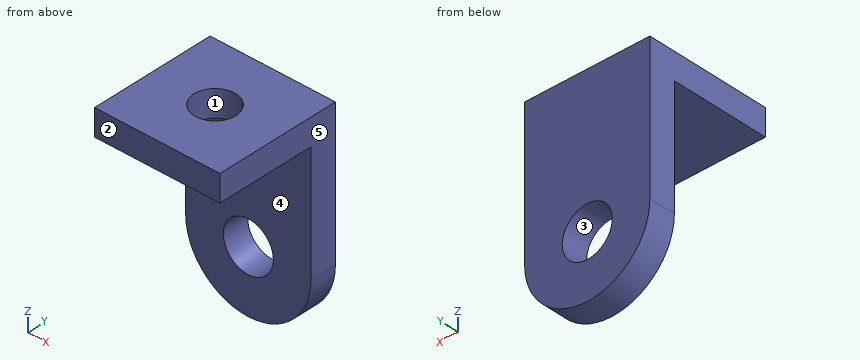
```python
from build123d import *

# Parameters (mm, degrees)
SKETCH1_W           = 15
SKETCH1_H           = 15
SKETCH1_R           = 2.5
BOSS_EXTRUDE1_DEPTH = 3.175
SKETCH2_R           = 3
BOSS_EXTRUDE2_DEPTH = 3.175


with BuildPart() as part:
    # Sketch1 → Boss-Extrude1 (new body)
    with BuildSketch(Plane.XY):
        with Locations((0, -7.5)):
            Rectangle(SKETCH1_W, SKETCH1_H)
        with Locations((0, -7.5)):
            Circle(SKETCH1_R, mode=Mode.SUBTRACT)
    extrude(amount=BOSS_EXTRUDE1_DEPTH)

    # Sketch2 → Boss-Extrude2 (add)
    with BuildSketch(Plane(origin=(0, 0, 0), x_dir=(1, 0, 0), z_dir=(0, 1, 0))):
        with BuildLine():
            Line((-7.5, 14.26), (-7.5, 0))
            Line((-7.5, 0), (7.5, 0))
            Line((7.5, 0), (7.5, 14.26))
            ThreePointArc((7.5, 14.26), (0, 21.76), (-7.5, 14.26))
        make_face()
        with Locations(Location((0, 14.26, 0), (0, 0, 270))):
            Circle(SKETCH2_R, mode=Mode.SUBTRACT)
    extrude(amount=-BOSS_EXTRUDE2_DEPTH)


solid = part.part
```
Input: part model. Units: mm. Frame: model coordinates. Face numbers are marked on the shaded views. A direction names the side the tool comes from. Give positions to 0.01 mm unless a question says otherwise; leave off trailing zeros. Order: outer loops, then holes, each group sorted by start corner. A loop starts at its lowest first (then second) coordinate and runs counter-clockwise, first axis right, second up.
1. Cut plane A-A (x = 0). Return loops of the section in (y, z) (3 decimals).
Computed:
outline: (-15, 0) - (-10, 0) - (-10, 3.175) - (-15, 3.175) - close; (-5, 0) - (-3.175, 0) - (-3.175, -11.26) - (0, -11.26) - (0, 3.175) - (-5, 3.175) - close; (-3.175, -21.76) - (0, -21.76) - (0, -17.26) - (-3.175, -17.26) - close
2. Set-up query: the marked faces 4 and 5. Return all of +Z, -Z, +X, -X, +Y, -Y with unobstructed straight access to the full face (end or side cutting, diameter ignored); none if empty.
Computed:
face 4: -Z, +X, -X, -Y
face 5: +Z, -Z, +X, +Y, -Y
3. Cut plane C-C (y = -2.75). Return loops of the section in (x, z) (3 decimals).
Computed:
outline: (-7.5, -14.26) arc R7.5 ccw to (7.5, -14.26) - (7.5, 3.175) - (-7.5, 3.175) - close; hole circle Ø6 at (0, -14.26)
4. Cut plane B-B (y = -5.5). Return loops of the section in (x, z) (3 decimals), and give its area (3 significant figures).
Computed:
outline: (-7.5, 0) - (-1.5, 0) - (-1.5, 3.175) - (-7.5, 3.175) - close; (1.5, 0) - (7.5, 0) - (7.5, 3.175) - (1.5, 3.175) - close
area: 38.1 mm2
5. Pin query (flat end, axial travel): pin 1 Ø3 at (x, z) = (0, -9.5) entering from -Y (3 decimals); pin 2 Ø3.5 at (x, y) = (2.5, -11) entering from -Z. Return the tip coordinate at first contact, or that it passes through.
Computed:
pin 1: stops at y = -3.175
pin 2: stops at z = 0
6. Draft query along Y for the marked faces 1, 2 and 3. Return one class per face: released by +Y, released by -Y, zero draft, split by the parting line, or undercut.
Computed:
face 1: undercut
face 2: released by -Y
face 3: zero draft
7. Cut plane D-D (x = -6). Return loops of the section in (y, z) (3 decimals).
Computed:
outline: (-15, 0) - (-3.175, 0) - (-3.175, -18.76) - (0, -18.76) - (0, 3.175) - (-15, 3.175) - close
8. Line query: probe 1 along X at (y, z) = (-2.3, -14.26); probe 2 along Y at (x, z) = (0, 1.5); probe 3 along Y at (x, z) = (-5.5, -0.25) (3 decimals). Output: solid intervals per line, ascending.
Computed:
probe 1: x = -7.5 to -3, 3 to 7.5
probe 2: y = -15 to -10, -5 to 0
probe 3: y = -3.175 to 0
